Here's how the part is built. I have some questions about the finished solid (model axes, mm). Face numbers are marked on the shaded views. A direction names the side the tool comes from. Give positions to 0.01 mm unless a question says otherwise; leave off trailing zeros. Loops run counter-clockwise (first coordinate to the right, second up) from the corner with the lowest first, then second, coordinate; pieces in that order, holes last.
Q1. Thinking about a two-plate mould opening in X: for the marked faces 1, 2 and 3, which applies, pulls with the +X half, pulls with the -X half, needs draft (parallel to the pull), parting line crosses it, or undercut?
Q2. I need wall thicknesses on probe 1 along Y at (x, z) = (1.15, -1.85); probe 2 along X at (y, z) = (27, -1.5); probe 3 along X at (y, z) = (17.5, -1.6). Which ranges of each line are inside material? Lowest first, please.
Q3. Suppose I cut it at B-B (y = 7). List the corners of the cut face in (x, z) for me, and give its area (3 significant figures).
Q4. Suppose I cut it at C-C (x = -0.6). List the corners of the cut face in (y, z) for me, and give its area (3 significant figures).
Q5. Suppose I cut it at A-A (z = 0). List the corners of the cut face in (x, y) for me, and give its area (3 significant figures).
Q6. Suppose I cut it at D-D (z = -1.85). List the corners of the cut face in (x, y) for me, and give its area (3 significant figures).
Q7. For the marked faces 4, 5 and 6, which set-ups out of +Z, -Z, +X, -X, +Y, -Y let a thin tool reach every point of the face, with its end or its side?
```python
from build123d import *

# Parameters (mm, degrees)
BOSS_EXTRUDE1_DEPTH = 30
SKETCH3_R           = 1.42
BOSS_EXTRUDE2_DEPTH = 3
BOSS_EXTRUDE3_START = 3
SKETCH4_R           = 1.42
BOSS_EXTRUDE3_DEPTH = 3


with BuildPart() as part:
    # Sketch2 → Boss-Extrude1 (new body)
    with BuildSketch(Plane(origin=(0, 0, 0), x_dir=(1, 0, 0), z_dir=(0, 1, 0))):
        Polygon((0, 2.886751346), (-2.5, 1.443375673), (-2.5, -1.443375673), (0, -2.886751346), (2.5, -1.443375673), (2.5, 1.443375673), align=None)
    extrude(amount=BOSS_EXTRUDE1_DEPTH)

    # Sketch3 → Boss-Extrude2 (add)
    with BuildSketch(Plane(origin=(0, 30, 0), x_dir=(1, 0, 0), z_dir=(0, 1, 0))):
        with Locations(Location((0, 0, 0), (0, 0, 270))):
            Circle(SKETCH3_R)
    extrude(amount=BOSS_EXTRUDE2_DEPTH)

    # Sketch4 → Boss-Extrude3 (add)
    with BuildSketch(Plane(origin=(0, 0, 0), x_dir=(-1, 0, 0), z_dir=(0, -1, 0)).offset(BOSS_EXTRUDE3_START)):
        with Locations(Location((0, 0, 0), (0, 0, 270))):
            Circle(SKETCH4_R)
    extrude(amount=-BOSS_EXTRUDE3_DEPTH)


solid = part.part
```
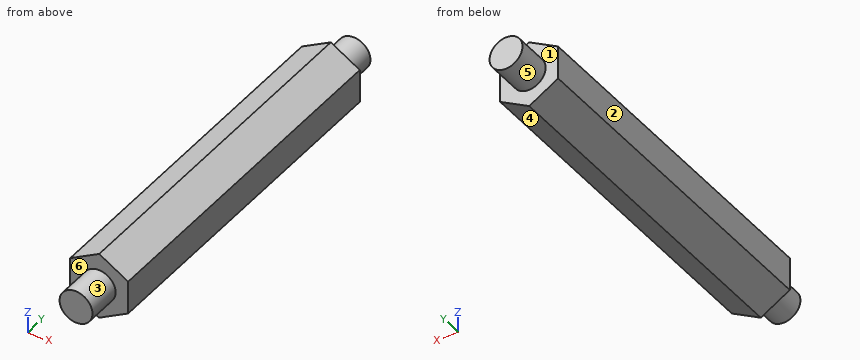
Solutions:
1. face 1: needs draft
1. face 2: pulls with the -X half
1. face 3: parting line crosses it
2. probe 1: y = 0 to 30
2. probe 2: x = -2.4 to 2.4
2. probe 3: x = -2.23 to 2.23
3. outline: (-2.5, -1.44) - (0, -2.89) - (2.5, -1.44) - (2.5, 1.44) - (0, 2.89) - (-2.5, 1.44) - close
3. area: 21.7 mm2
4. outline: (-3, -1.29) - (0, -1.29) - (0, -2.54) - (30, -2.54) - (30, -1.29) - (33, -1.29) - (33, 1.29) - (30, 1.29) - (30, 2.54) - (0, 2.54) - (0, 1.29) - (-3, 1.29) - close
4. area: 168 mm2
5. outline: (-2.5, 0) - (-1.42, 0) - (-1.42, -3) - (1.42, -3) - (1.42, 0) - (2.5, 0) - (2.5, 30) - (1.42, 30) - (1.42, 33) - (-1.42, 33) - (-1.42, 30) - (-2.5, 30) - close
5. area: 167 mm2
6. outline: (-1.8, 0) - (1.8, 0) - (1.8, 30) - (-1.8, 30) - close
6. area: 108 mm2
7. face 4: -Z, +X, +Y, -Y
7. face 5: +Y
7. face 6: -Y
